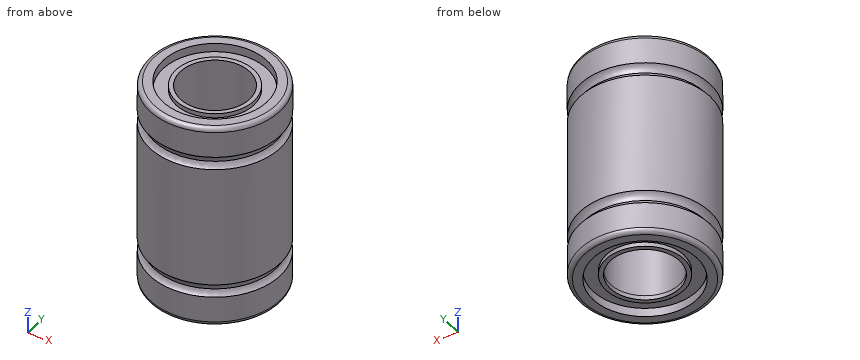
Autodesk Inventor part; units mm, degrees
ref_plane "YZ Plane" through (0, 0, 0) normal (1, 0, 0) x (0, 1, 0)
ref_plane "XZ Plane" through (0, 0, 0) normal (0, 1, 0) x (-1, 0, 0)
ref_plane "XY Plane" through (0, 0, 0) normal (0, 0, 1) x (1, 0, 0)
sketch "Sketch1" plane through (0, 0, 0) normal (0, 0, 1) x (1, 0, 0)
  circle A0 centre (0, 0) radius 4
  circle A1 centre (0, 0) radius 6
  dimension "d0" = 8
  dimension "d2" = 12
sketch "Sketch1 outline for Extrusion1" plane through (0, 0, 0) normal (0, 0, 1) x (1, 0, 0)
  circle A0 centre (0, 0) radius 6
  circle A1 centre (0, 0) radius 4
extrude "Extrusion1" add sketch "Sketch1 outline for Extrusion1" along normal blind 22
sketch "Sketch2" plane through (0, 0, 22) normal (0, 0, 1) x (1, 0, 0)
  circle A0 centre (0, 0) radius 6
  circle A1 centre (0, 0) radius 7.5
  dimension "d5" = 15
sketch "Sketch2 outline for Extrusion2" plane through (0, 0, 22) normal (0, 0, 1) x (1, 0, 0)
  circle A0 centre (0, 0) radius 7.5
  circle A1 centre (0, 0) radius 6
extrude "Extrusion2" add sketch "Sketch2 outline for Extrusion2" along normal blind 1 and the other way blind 2.5
sketch "Sketch3" plane through (0, 0, 19.5) normal (0, 0, -1) x (-1, 0, 0)
  circle A0 centre (0, 0) radius 6
  circle A1 centre (0, 0) radius 7.5
  circle A2 centre (0, 0) radius 7
  dimension "d11" = 14
sketch "Sketch3 outline for Extrusion3" plane through (0, 0, 19.5) normal (0, 0, -1) x (-1, 0, 0)
  circle A0 centre (0, 0) radius 7
  circle A1 centre (0, 0) radius 6
extrude "Extrusion3" add sketch "Sketch3 outline for Extrusion3" along normal blind 1.5
sketch "Sketch4" plane through (0, 0, 18) normal (0, 0, -1) x (-1, 0, 0)
  circle A0 centre (0, 0) radius 6
  circle A1 centre (0, 0) radius 7
  circle A2 centre (0, 0) radius 7.5
  dimension "d15" = 15
sketch "Sketch4 outline for Extrusion4" plane through (0, 0, 18) normal (0, 0, -1) x (-1, 0, 0)
  circle A0 centre (0, 0) radius 7.5
  circle A1 centre (0, 0) radius 6
extrude "Extrusion4" add sketch "Sketch4 outline for Extrusion4" along normal blind 14
sketch "Sketch5" plane through (0, 0, 4) normal (0, 0, -1) x (-1, 0, 0)
  circle A0 centre (0, 0) radius 6
  circle A1 centre (0, 0) radius 7.5
  circle A2 centre (0, 0) radius 7
  dimension "d19" = 14
sketch "Sketch5 outline for Extrusion5" plane through (0, 0, 4) normal (0, 0, -1) x (-1, 0, 0)
  circle A0 centre (0, 0) radius 7
  circle A1 centre (0, 0) radius 6
extrude "Extrusion5" add sketch "Sketch5 outline for Extrusion5" along normal blind 1.5
sketch "Sketch6" plane through (0, 0, 2.5) normal (0, 0, -1) x (-1, 0, 0)
  circle A0 centre (0, 0) radius 6
  circle A1 centre (0, 0) radius 7
  circle A2 centre (0, 0) radius 7.5
  dimension "d23" = 15
sketch "Sketch6 outline for Extrusion6" plane through (0, 0, 2.5) normal (0, 0, -1) x (-1, 0, 0)
  circle A0 centre (0, 0) radius 7.5
  circle A1 centre (0, 0) radius 6
extrude "Extrusion6" add sketch "Sketch6 outline for Extrusion6" along normal blind 3.5
fillet "Fillet1" radius 1 4 edges at (7, 0, 19.5) (7, 0, 4) (7, 0, 2.5) (7, 0, 18)
fillet "Fillet2" radius 0.5 2 edges at (-7.5, 0, 23) (7.5, 0, -1)
sketch "Sketch7" plane through (0, 0, 22) normal (0, 0, 1) x (1, 0, 0)
  circle A0 centre (0, 0) radius 4
  circle A1 centre (0, 0) radius 6
  circle A2 centre (0, 0) radius 4.5
  dimension "d29" = 9
sketch "Sketch7 outline for Extrusion7" plane through (0, 0, 22) normal (0, 0, 1) x (1, 0, 0)
  circle A0 centre (0, 0) radius 4.5
  circle A1 centre (0, 0) radius 4
extrude "Extrusion7" add sketch "Sketch7 outline for Extrusion7" along normal blind 0.5
sketch "Sketch8" plane through (0, 0, 0) normal (0, 0, -1) x (-1, 0, 0)
  circle A0 centre (0, 0) radius 4
  circle A1 centre (0, 0) radius 6
  circle A2 centre (0, 0) radius 4.5
  dimension "d34" = 9
sketch "Sketch8 outline for Extrusion8" plane through (0, 0, 0) normal (0, 0, -1) x (-1, 0, 0)
  circle A0 centre (0, 0) radius 4.5
  circle A1 centre (0, 0) radius 4
extrude "Extrusion8" add sketch "Sketch8 outline for Extrusion8" along normal blind 0.5
properties part number "lineair bearing 8 x15 x 24"
Source: CAD feature listing. Evaluate the final solid. Frame: model axes, mm. Coordinates: 2 decimals unless noted, no trailing zeros. Write each loop counter-clockwise with the first axis right and the second up, starting at its lowest first coordinate (ties: lowest second). Pieces come first, ordered by that corner, then holes. Notation, with made-up numbers: (0, 13.5) - (55, 13.5) arc R34 cw to (55, 50.5) - close; hole circle Ø5 at (63.25, -35). An arc over 180 degrees is marked (long way). Answer as a JSON object with one key per item and string values.
Q1. Section query A-A, the plane z = 5. Output: boundary loops of the cut face in (x, y).
Ans:
{"outline": "circle Ø15 at (0, 0); hole circle Ø8 at (0, 0)"}
Q2. Material intervals for line 1 (Y direction, x = 0, z = -0.2); line 2 (Z direction, x = -1.75, y = 7); line 3 (Z direction, x = 3.5, y = 4), sorted ascending. Write a range as [from, to].
Ans:
{"line 1": "y = [-7.5, -6], [-4.5, -4], [4, 4.5], [6, 7.5]", "line 2": "z = [-0.95, 2.73], [3.75, 18.23], [19.25, 22.95]", "line 3": "z = [0, 22]"}
Q3. First-contact query: pin 1 Ø5 at (y, z) = (-1, 5.5) entering from -X; pin 2 Ø6 at (x, y) = (-0.5, 2) entering from +Z; pin 3 Ø2.5 at (x, y) = (1, -2) entering from -Z. Flat tips, straight axial feed; report the tip coordinate or a pass-through.
Ans:
{"pin 1": "stops at x = -7.5", "pin 2": "stops at z = 22.5", "pin 3": "passes through"}
